The listing builds one solid part. Answer for the finished solid, in the listing's coordinates (mm). A direction names the side the tool comes from. Give positions to 0.01 mm unless a question says otherwise; leave off trailing zeros. Order: outer loops, then holes, each group sorted by start corner. A loop starts at its lowest first (then second) coordinate and runs counter-clockwise, first axis right, second up.
```python
from build123d import *

# Parameters (mm, degrees)
SKETCH_2_R          = 2.5
SKETCH_2_R_2        = 1.65
EXTRUDE_1_DEPTH     = 5
SKETCH_3_W          = 5
SKETCH_3_H          = 7.033503338
EXTRUDE_2_DEPTH     = 40
CUT_EXTRUDE_1_REACH = 7
SKETCH_6_W          = 30
SKETCH_6_H          = 63
CUT_EXTRUDE_2_DEPTH = 10
FILLET_1_R          = 6
FILLET_2_R          = 2
FILLET_3_R          = 1


with BuildPart() as part:
    # 草图2 → 凸台-拉伸1 (new body)
    with BuildSketch(Plane.XY):
        with BuildLine():
            Line((90, -2.836370327), (90, -0.033503338))
            Line((90, -0.033503338), (90, 7.163629673))
            Line((90, 7.163629673), (70.37335416, 7.163629673))
            Line((70.37335416, 7.163629673), (70.37335416, 47.663629673))
            Line((70.37335416, 47.663629673), (90, 47.663629673))
            Line((90, 47.663629673), (90, 55.071074042))
            Line((90, 55.071074042), (56.86982625, 91.020052584))
            Line((56.86982625, 91.020052584), (68.87304018, 91.020052584))
            ThreePointArc((68.87304018, 91.020052584), (71.37304018, 93.520052584), (68.87304018, 96.020052584))
            Line((68.87304018, 96.020052584), (52.261882562, 96.020052584))
            Line((52.261882562, 96.020052584), (36.613354259, 113))
            Line((36.613354259, 113), (0, 113))
            Line((0, 113), (0, 0))
            Line((0, 0), (0, -2.836370327))
            Line((0, -2.836370327), (90, -2.836370327))
        make_face()
        Polygon((5, 7.033503338), (5, 44.840982038), (50.37304018, 7.033503338), (10, 7.033503338), align=None, mode=Mode.SUBTRACT)
        Polygon((60.37304018, 7.033503338), (14.814475837, 47.663629673), (60.37304018, 47.663629673), align=None, mode=Mode.SUBTRACT)
        with Locations((75.24372976, 3.308629673)):
            Circle(SKETCH_2_R, mode=Mode.SUBTRACT)
        with Locations((85.24372976, 3.308629673)):
            Circle(SKETCH_2_R, mode=Mode.SUBTRACT)
        with Locations((75.24372976, 51.518629673)):
            Circle(SKETCH_2_R, mode=Mode.SUBTRACT)
        with Locations((85.24372976, 51.518629673)):
            Circle(SKETCH_2_R, mode=Mode.SUBTRACT)
        Polygon((5, 106.225949783), (31, 106.225949783), (31, 54.840982038), (11.37304018, 54.840982038), (6.37304018, 54.840982038), (5, 54.840982038), (5, 91.020052584), (5, 96.020052584), align=None, mode=Mode.SUBTRACT)
        with Locations((38.87304018, 57.520052584)):
            Circle(SKETCH_2_R_2, mode=Mode.SUBTRACT)
        with Locations((38.87304018, 93.520052584)):
            Circle(SKETCH_2_R_2, mode=Mode.SUBTRACT)
        with BuildLine():
            Line((36.37304018, 106.587975229), (80.964081518, 58.203007486))
            Line((80.964081518, 58.203007486), (71.196585176, 58.203007486))
            ThreePointArc((71.196585176, 58.203007486), (68.87304018, 59.834918346), (66.549495185, 58.203007486))
            Line((66.549495185, 58.203007486), (63.373040182, 58.203007486))
            Line((63.373040182, 58.203007486), (60.53695685, 55.071074042))
            Line((60.53695685, 55.071074042), (41.37304018, 55.071074042))
            Line((41.37304018, 55.071074042), (41.342732423, 55.071074042))
            Line((41.342732423, 55.071074042), (41.342732423, 57.520052584))
            ThreePointArc((41.342732423, 57.520052584), (40.619376312, 59.266388716), (38.87304018, 59.989744826))
            Line((38.87304018, 59.989744826), (36.37304018, 59.989744826))
            Line((36.37304018, 59.989744826), (36.37304018, 91.020052584))
            Line((36.37304018, 91.020052584), (38.87304018, 91.020052584))
            ThreePointArc((38.87304018, 91.020052584), (41.37304018, 93.520052584), (38.87304018, 96.020052584))
            Line((38.87304018, 96.020052584), (36.37304018, 96.020052584))
            Line((36.37304018, 96.020052584), (36.37304018, 106.587975229))
        make_face(mode=Mode.SUBTRACT)
        with BuildLine():
            ThreePointArc((67.371017344, 58.203007486), (68.87304018, 59.170052584), (70.375063017, 58.203007486))
            ThreePointArc((70.375063017, 58.203007486), (70.485621602, 57.869453729), (70.52304018, 57.520052584))
            ThreePointArc((70.52304018, 57.520052584), (68.523639036, 55.907471163), (67.371017344, 58.203007486))
        make_face(mode=Mode.SUBTRACT)
        with Locations((68.87304018, 93.520052584)):
            Circle(SKETCH_2_R_2, mode=Mode.SUBTRACT)
    extrude(amount=EXTRUDE_1_DEPTH)

    # 草图3 → 凸台-拉伸2 (add)
    with BuildSketch(Plane(origin=(0, 0, 0), x_dir=(-1, 0, 0), z_dir=(0, 0, -1))):
        Polygon((0, -2.836370327), (0, 0), (-5, 0), (-90, 0), (-90, -2.836370327), align=None)
        with Locations((-2.5, 3.516751669)):
            Rectangle(SKETCH_3_W, SKETCH_3_H)
        Polygon((-5, 7.033503338), (0, 7.033503338), (0, 113), (-5, 113), (-5, 106.225949783), (-5, 54.840982038), (-5, 44.840982038), align=None)
    extrude(amount=EXTRUDE_2_DEPTH)

    # 草图6 → 切除-拉伸1 (cut, up to next)
    with BuildSketch(Plane(origin=(5, 0, 0), x_dir=(0, 0, -1), z_dir=(1, 0, 0)), mode=Mode.PRIVATE) as cut_extrude_1_sk1:
        with Locations((25, 41.5)):
            Rectangle(SKETCH_6_W, SKETCH_6_H)
    cut_extrude_1_tool1 = extrude(cut_extrude_1_sk1.sketch, amount=-CUT_EXTRUDE_1_REACH, mode=Mode.PRIVATE) & part.part
    add(cut_extrude_1_tool1.solids().sort_by_distance((5, 41.5, -25))[0], mode=Mode.SUBTRACT)

    # 草图7 → 切除-拉伸2 (cut)
    with BuildSketch(Plane(origin=(0, 0, 0), x_dir=(1, 0, 0), z_dir=(0, 1, 0))):
        Polygon((80, 40), (66, 26), (29, 26), (15, 40), align=None)
    extrude(amount=-CUT_EXTRUDE_2_DEPTH, mode=Mode.SUBTRACT)

    # 圆角1
    fillet_1_edges = [part.edges().sort_by_distance(p)[0] for p in [
        (90, -2.836370327, -17.5),
        (90, 55.071074042, 2.5),
        (36.613354259, 113, 2.5),
    ]]
    fillet(fillet_1_edges, radius=FILLET_1_R)

    # 圆角2
    fillet_2_edges = [part.edges().sort_by_distance(p)[0] for p in [
        (0, 73, -25),
        (0, 10, -25),
        (0, 41.5, -10),
        (5, 73, -25),
        (5, 41.5, -10),
        (5, 10, -25),
    ]]
    fillet(fillet_2_edges, radius=FILLET_2_R)

    # 圆角3
    fillet_3_edges = [part.edges().sort_by_distance(p)[0] for p in [
        (90, 47.663629673, 2.5),
        (90, 7.163629673, 2.5),
    ]]
    fillet(fillet_3_edges, radius=FILLET_3_R)


solid = part.part
```
1) Find section A-A (z = -31). Write down the section's boundary in (x, y), then the cut area to 3 significant figures.
Geometry says:
outline: (0, -2.84) - (24, -2.84) - (24, 0) - (5, 0) - (5, 8) arc R2 ccw to (3, 10) - (2, 10) arc R2 ccw to (0, 8) - close; (0, 75) arc R2 ccw to (2, 73) - (3, 73) arc R2 ccw to (5, 75) - (5, 113) - (0, 113) - close; (71, -2.84) - (84, -2.84) arc R6 ccw to (89.1, 0) - (71, 0) - close
area: 362 mm2
2) For a pull along Y with two mould halves and no side action, classify faces 1 (the cylindrical face through (40.638, 59.247, 2.465)), 2 (the flat face through (48, -1, -26)), 3 (the flat face through (46, 0, -15)), 4 (the flat face through (76, 58.203, 2)) as +Y half, -Y half, draft (parallel to the pull), parting line (faces both ways), or undercut.
Geometry says:
face 1: undercut
face 2: draft
face 3: +Y half
face 4: undercut
3) A tool of negligible diameter and unlimited length cuts with its end or side. For faces 5 (the flat face through (0, 67, -7)), 6 (the flat face through (65, 58.203, 2)), 7 (the flat face through (80, 47.664, 2)), 8 (the flat face through (61, 96.02, 2)), 9 (the flat face through (34, 56, 5)), from which of +Z, -Z, +X, -X, +Y, -Y can it reach the whole face along a straight path? Write none if from no direction.
Geometry says:
face 5: +Z, -Z, -X, +Y, -Y
face 6: +Z, -Z
face 7: +Z, -Z, +X
face 8: +Z, -Z, +X, +Y
face 9: +Z, +X, -X, +Y, -Y
4) Find section C-C (y = 13). Write down the section's boundary in (x, z), then the cut area to 3 significant figures.
Geometry says:
outline: (0, -8) arc R2 ccw to (2, -10) - (3, -10) arc R2 ccw to (5, -8) - (5, 5) - (0, 5) - close; (43.21, 0) - (53.68, 0) - (53.68, 5) - (43.21, 5) - close; (60.37, 0) - (70.37, 0) - (70.37, 5) - (60.37, 5) - close
area: 176 mm2
5) Find section B-B (z = -23.5). Write down the section's boundary in (x, y).
Geometry says:
outline: (0, -2.84) - (84, -2.84) arc R6 ccw to (89.1, 0) - (5, 0) - (5, 8) arc R2 ccw to (3, 10) - (2, 10) arc R2 ccw to (0, 8) - close; (0, 75) arc R2 ccw to (2, 73) - (3, 73) arc R2 ccw to (5, 75) - (5, 113) - (0, 113) - close
6) Straight lines are drawn through the part: probe 1 along X at (y, z) = (77, 1); probe 2 along Y at (x, z) = (21.5, 2.5); probe 3 along Y at (x, z) = (85.5, 1). For each, find the intervals that lie inside material, in ascending order.
Geometry says:
probe 1: x = 0 to 5, 31 to 36.37, 63.64 to 69.79
probe 2: y = -2.84 to 7.03, 31.09 to 41.7, 47.66 to 54.84, 106.23 to 113
probe 3: y = -2.65 to 0.82, 5.8 to 7.16, 47.66 to 49.03, 54.01 to 59.95
7) Find section D-D (y = 41). Write down the section's boundary in (x, z), then the cut area to 3 significant figures.
Geometry says:
outline: (0, -8) arc R2 ccw to (2, -10) - (3, -10) arc R2 ccw to (5, -8) - (5, 5) - (0, 5) - close; (9.61, 0) - (22.29, 0) - (22.29, 5) - (9.61, 5) - close; (60.37, 0) - (70.37, 0) - (70.37, 5) - (60.37, 5) - close
area: 187 mm2
8) Given P1, Ø3, axis at x = 85.24, y = 51.52, coming from the +Z side; P2, Ø2.5, axis at x = 65, z = 3, coming from the +Y side; P3, Ø2.5, axis at y = 100.5, z = 2, coming from the +X side; P4, Ø4, axis at x = 75, z = -1, coming from the +Y side, each flat-ended and moving along its own axis, determine where each tip first touches the part or whether it passes through.
Geometry says:
P1: passes through
P2: stops at y = 96.02
P3: stops at x = 49.29
P4: stops at y = 73.23
